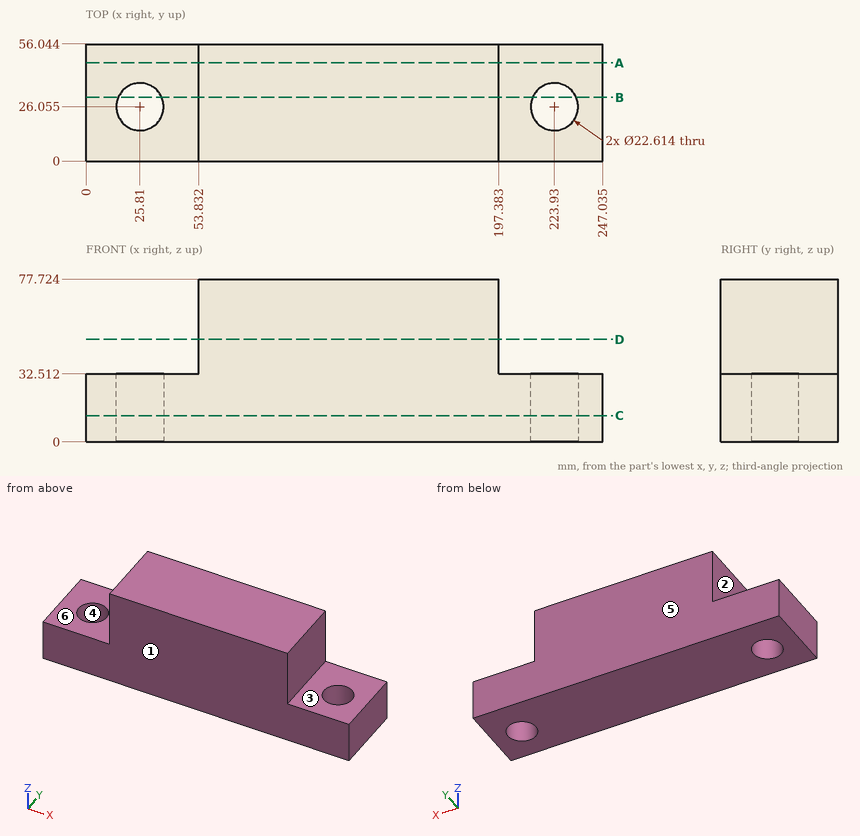
Source: three-view drawing plus pictorial views. Frame: mm from the lowest corner of the part. A direction names the side the tool comes from. Round coordinates to 2 decimals unless told otherwise and drop trailing zeros. Loops run counter-clockwise (first coordinate to the right, second up) from the corner with the lowest first, then second, coordinate; pieces in that order, holes last.
Q1. Section A-A on y = 47. Return loops of the section in (x, z) (1 decimal).
Q2. Pin query (flat end, axial travel): P1, Ø1, axis at y = 7.5, z = 35, coming from the -X side; P2, Ø8, axis at y = 44, z = 63.5, coming from the +X side; P3, Ø25, axis at x = 212.5, y = 25, coming from the +Z side. Return the tip coordinate at first contact, or that it passes through.
Q3. Section D-D on z = 49. Return loops of the section in (x, y).
Q4. Access query for the marked faces 1, 2 and 3. Directions: +Z, -Z, +X, -X, +Y, -Y. A direction counts if a zero-diameter tool reaches every point of the face in a straight line with its end or side. Return the directions, or none.
Q5. Material intervals for L1, parallel to X at y = 23, z = 23 (1 decimal); L2, parallel to Z at x = 200.5, y = 41.5; L3, parallel to X at y = 37, z = 50, sorted ascending.
Q6. Pull-direction query (Y, two-part tool) for the marked faces 4, 5 and 6; classes: released by +Y, released by -Y, zero draft, split by the parting line, or undercut.
Q7. Section C-C on z = 12.5. Return loops of the section in (x, y) (1 decimal).
Q8. Section B-B on y = 30.5. Return loops of the section in (x, z) (1 decimal).
Evaluation:
1. outline: (0, 0) - (247, 0) - (247, 32.5) - (197.4, 32.5) - (197.4, 77.7) - (53.8, 77.7) - (53.8, 32.5) - (0, 32.5) - close
2. P1: stops at x = 53.83
2. P2: stops at x = 197.38
2. P3: stops at z = 32.51
3. outline: (53.83, 0) - (197.38, 0) - (197.38, 56.04) - (53.83, 56.04) - close
4. face 1: +Z, -Z, +X, -X, -Y
4. face 2: +Z, -X, +Y, -Y
4. face 3: +Z, +X, +Y, -Y
5. L1: x = 0 to 14.9, 36.7 to 213, 234.8 to 247
5. L2: z = 0 to 32.51
5. L3: x = 53.83 to 197.38
6. face 4: undercut
6. face 5: released by +Y
6. face 6: zero draft
7. outline: (0, 0) - (247, 0) - (247, 56) - (0, 56) - close; hole circle Ø22.6 at (25.8, 26.1); hole circle Ø22.6 at (223.9, 26.1)
8. outline: (0, 0) - (15.4, 0) - (15.4, 32.5) - (0, 32.5) - close; (36.2, 0) - (213.5, 0) - (213.5, 32.5) - (197.4, 32.5) - (197.4, 77.7) - (53.8, 77.7) - (53.8, 32.5) - (36.2, 32.5) - close; (234.3, 0) - (247, 0) - (247, 32.5) - (234.3, 32.5) - close
